Could you check a few things on this model? Use its own coordinates, in mm. A direction names the side the tool comes from. Round coordinates to 2 decimals unless told otherwise and drop trailing zeros. Loops run counter-clockwise (first coordinate to the right, second up) from the corner with the lowest first, then second, coordinate; pieces in that order, holes last. Notation, with made-up numbers: (3, -17) -> (49, -17) arc R18 ccw to (49, -11) -> close; hole circle Ø2 at (-38, 6.5). An arc over 180 degrees is marked (long way). One line per item, written item: value.
Autodesk Inventor part; units mm, degrees
ref_plane "YZ Plane" through (0, 0, 0) normal (1, 0, 0) x (0, 1, 0)
ref_plane "XZ Plane" through (0, 0, 0) normal (0, 1, 0) x (-1, 0, 0)
ref_plane "XY Plane" through (0, 0, 0) normal (0, 0, 1) x (1, 0, 0)
sketch "Sketch1" plane through (0, 0, 0) normal (0, 0, 1) x (1, 0, 0)
  arc A0 (0.4294, -77.1903) -> (350.3978, -24.4313) centre (0.4294, 1109.9183) ccw
  arc A1 (0.2037, -92.1903) -> (354.8199, -38.7647) centre (0.4294, 1109.9183) ccw
  line L0 (0.2076, -71.1704) -> (0.2037, -92.1903)
  line L1 (350.3978, -24.4313) -> (372.3, -24.4313) construction
  line L2 (0, 0) -> (375, 0)
  line L3 (375, 0) -> (375, -16.8411)
  line L4 (350.3978, -24.4313) -> (375, -16.8411)
  line L5 (354.8199, -38.7647) -> (363.9727, -35.9408)
  line L6 (375, -16.8411) -> (363.9727, -35.9408)
  line L7 (375, -16.8411) -> (397.0545, -16.8411) construction
  arc A2 (-349.9649, -24.2998) -> (0.4294, -77.1903) centre (0.4294, 1109.9183) ccw
  arc A3 (-354.3924, -38.6315) -> (0.2037, -92.1903) centre (0.4294, 1109.9183) ccw
  line L8 (-349.9649, -24.2998) -> (-374.5643, -16.7003)
  line L9 (-354.3924, -38.6315) -> (-363.5442, -35.8042)
  line L10 (-374.5643, -16.7003) -> (-363.5442, -35.8042)
  arc A4 (0.4294, -107.1903) -> (359.242, -53.098) centre (0.4294, 1109.9183) ccw
  line L11 (359.242, -53.098) -> (374.0198, -48.5388)
  line L12 (374.0198, -48.5388) -> (388.2749, -23.8483)
  line L13 (363.9727, -35.9408) -> (0.4294, -35.9408)
  point P0 (350.1634, -39.5425)
  point P1 (287.1787, -57.4891)
  dimension "d0" = 15
  dimension "d12" = 375
  dimension "d13" = 120
  dimension "d15" = 15
  dimension "d16" = 363.5433
extrude "Extrusion1" add sketch "Sketch1" along normal blind 30
sketch "Sketch2" plane through (0, 0, 0) normal (0, 1, 0) x (-1, 0, 0)
  line L0 (0, 0) -> (0, 15)
  circle A0 centre (0, 15) radius 5
  dimension "d5" = 15
  dimension "d6" = 10
extrude "Extrusion2" cut sketch "Sketch2" against normal blind 300
fillet "Fillet5" radius 3 17 edges at (359.3963, -37.3527, 30) (-358.9683, -37.2179, 30) (179.5153, -78.7757, 30) (-358.9683, -37.2179, 0) (359.3963, -37.3527, 0) (179.5153, -78.7757, 0) (-363.5442, -35.8042, 15) (-369.0543, -26.2523, 30) (-362.2646, -20.5001, 30) (362.6989, -20.6362, 30) (-176.7524, -63.8932, 30) (-369.0543, -26.2523, 0) (-374.5643, -16.7003, 15) (369.4864, -26.3909, 0) (363.9727, -35.9408, 15) (369.4864, -26.3909, 30) (375, -16.8411, 15)
properties part number "leaf 2" material "Steel, Carbon"
Item 1: Will these pins go through, and if not, where does the flat tip stop? pin 1 Ø6 at (y, z) = (-29.5, 17.5) entering from -X; pin 2 Ø12 at (y, z) = (-38.5, 15.5) entering from +X; pin 3 Ø4 at (x, z) = (-276, 15.5) entering from +Y.
Output:
pin 1: stops at x = -368.91
pin 2: stops at x = 365.96
pin 3: stops at y = -44.08
Item 2: For faces 1 (the face through (-174.29, -64.262, 13.311)), 2 (the face through (-29, -77, 0)), which set-ups out of +Z, -Z, +X, -X, +Y, -Y let a thin tool reach every point of the face, with its end or its side?
Output:
face 1: +Z, -Z, +Y
face 2: -Z, +X, -X, +Y, -Y
Item 3: I need wall thicknesses on line 1 (Z direction, x = 0, y = -84.25); line 2 (Y direction, x = 9, z = 14.5); line 3 (Z direction, x = -263, y = -61.5). Which ranges of each line are inside material? Lowest first, please. Write a range as from..to.
Output:
line 1: z = 0..10, 20..30
line 2: y = -92.16..-77.16
line 3: z = 0.44..29.56
Item 4: If we section it at A-A on z = 15: List the corners of the cut face in (x, y) for me.
Output:
outline: (-370.74, -23.32) -> (-364.13, -34.78) arc R3 ccw to (-362.42, -36.15) -> (-354.39, -38.63) arc R1202.11 ccw to (-5, -92.18) -> (-5, -77.18) arc R1187.11 cw to (-349.96, -24.3) -> (-367.26, -18.96) arc R3 ccw to start; (5, -92.18) arc R1202.11 ccw to (354.82, -38.76) -> (362.85, -36.29) arc R3 ccw to (364.56, -34.92) -> (371.18, -23.46) arc R3 ccw to (367.7, -19.09) -> (350.4, -24.43) arc R1187.11 cw to (5, -77.18) -> close
Item 5: If we mould it in two halves opening along X, with no side actions, what happens to faces 3 (the face through (-2, -83, 30)), 4 (the face through (-176.611, -79.082, 14.832)), 5 (the face through (179.849, -63.553, 13.311))? For each: released by +X, released by -X, zero draft, split by the parting line, or undercut.
Output:
face 3: zero draft
face 4: released by -X
face 5: undercut
